CAD build for the part. Positions are in the model's coordinates, mm. Coordinates: 2 decimals unless noted, no trailing zeros. Order: outer loops, then holes, each group sorted by start corner. A loop starts at its lowest first (then second) coordinate and runs counter-clockwise, first axis right, second up. Notation, with made-up numbers: (28, -13.5) - (61, -13.5) arc R17 cw to (61, 19.5) - close; hole circle Ø2 at (4.25, 24.5). An arc over 180 degrees is marked (long way). Write each question's results on one line, items separated by ' | '. Start each with the question number.
Q1. Wall check: probe 1 along Z at (x, y) = (-81, -0.9); probe 2 along Z at (x, y) = (0, -1.25); probe 3 along X at (y, z) = (-0.85, 132). Give the ranges that are in metal, low to high.
Q2. Pin check, flat tips, straight feed: P1, Ø2.5, axis at x = 24.87, z = 21.07, coming from the +Y side; P2, Ø1.6, axis at y = -2.5, z = -1, coming from the +X side; P3, Ø1.1, axis at x = -4, y = -2.5, coming from the -Z side. Stop position of each tip, or through.
Q3. Band-saw the part on B-B, the plane x = 74.5. Write the cut outline in (y, z).
Q4. Pull direction X, two halves, no side cores. Call faces 1 (the flat face through (161.809, -1.878, 105.064)), 2 (the flat face through (58, -3.81, 54)), 3 (the flat face through (155.96, -1.88, 7.79)): released by +X, released by -X, zero draft, split by the parting line, or undercut.
Q5. Band-saw the part on A-A, the plane y = -0.9. Count the separate pieces of the cut face and the enclosed holes in it, then the cut area to 3 significant figures.
```python
from build123d import *

# Parameters (mm, degrees)
F0_R     = 1.5875
F1_DEPTH = 3.81


with BuildPart() as f1:
    # F0 (on Front) → F1 (new body)
    with BuildSketch(Plane.XZ):
        with BuildLine():
            Line((-43.090851702, -3.1242), (-43.090851702, 0))
            Line((-43.090851702, 0), (11.7375096306, 0))
            Line((11.7375096306, 0), (45.617762953, 11.4486236125))
            add(Edge.make_bspline(
                [(45.617762953, 11.4486236125), (43.9961000977, 8.6191003913), (40.3730056188, 4.577922731), (44.1195508196, 1.4224311064), (45.617762953, 0)],
                knots=[0, 0, 0, 0, 0.5388146408, 1, 1, 1, 1], degree=3))
            Line((45.617762953, 0), (77.7362398488, 0))
            Line((77.7362398488, 0), (77.7362398488, -3.1242))
            Line((77.7362398488, -3.1242), (103.1362398488, -3.1242))
            Line((103.1362398488, -3.1242), (103.1362398488, 0))
            Line((103.1362398488, 0), (137.1024620031, 0))
            Line((137.1024620031, 0), (175.3601329191, 15.8024989069))
            add(Edge.make_bspline(
                [(176.9877400097, 108.5755596732), (171.7473141945, 103.3597046798), (164.3550587217, 79.2093285896), (191.2164116111, 47.498469968), (169.6077040725, 23.5923640125), (175.3601329191, 15.8024989069)],
                knots=[0, 0, 0, 0, 0.3117132351, 0.6730053796, 1, 1, 1, 1], degree=3))
            Line((176.9877400097, 108.5755596732), (146.1987151904, 101.452911742))
            ThreePointArc((146.1987151904, 101.452911742), (91.5320388396, 140.0844195098), (36.3692378486, 102.1647111449))
            add(Edge.make_bspline(
                [(-15.078710516, 63.5241562685), (0.3297940237, 63.5041378405), (27.1279570327, 77.8387740817), (31.1426373051, 91.6452955028), (36.3692378486, 102.1647111449)],
                knots=[0, 0, 0, 0, 0.5551499724, 1, 1, 1, 1], degree=3))
            add(Edge.make_bspline(
                [(-15.078710516, 63.5241562685), (-30.8021855302, 63.8675037628), (-65.4962545936, 70.9878737096), (-114.1797542997, 45.7754396965), (-122.9711554478, 12.7121701485), (-144.690851702, 0)],
                knots=[0.2992076009, 0.2992076009, 0.2992076009, 0.2992076009, 0.50107299, 0.7437623527, 1, 1, 1, 1], degree=3))
            Line((-144.690851702, 0), (-68.490851702, 0))
            Line((-68.490851702, 0), (-68.490851702, -3.1242))
            Line((-68.490851702, -3.1242), (-43.090851702, -3.1242))
        make_face()
        with Locations((-80.1899433136, 10.7241785154)):
            Circle(F0_R, mode=Mode.SUBTRACT)
        with Locations((-45.4173433136, 19.2251093046)):
            Circle(F0_R, mode=Mode.SUBTRACT)
        with Locations((-20.6142470102, 17.4490999235)):
            Circle(F0_R, mode=Mode.SUBTRACT)
        with Locations((0, 21.0686270148)):
            Circle(F0_R, mode=Mode.SUBTRACT)
        with Locations((24.8666, 21.0686270148)):
            Circle(F0_R, mode=Mode.SUBTRACT)
        with Locations((139.4535154104, 10.7241785154)):
            Circle(F0_R, mode=Mode.SUBTRACT)
        with BuildLine():
            ThreePointArc((30.7592003997, 41.2713398651), (30.8999876678, 40.90769576), (30.9478799796, 40.5207016819))
            ThreePointArc((30.9478799796, 40.5207016819), (27.8207722914, 40.1337076037), (30.7592003997, 41.2713398651))
        make_face(mode=Mode.SUBTRACT)
        with BuildLine():
            ThreePointArc((65.9967244268, 59.3286920018), (64.796218505, 57.7890843136), (63.0104040067, 58.5780538185))
            ThreePointArc((63.0104040067, 58.5780538185), (63.5221237134, 60.6452057975), (65.6301646769, 60.3433156541))
            ThreePointArc((65.6301646769, 60.3433156541), (65.9022748106, 59.8680961189), (65.9967244268, 59.3286920018))
        make_face(mode=Mode.SUBTRACT)
        with BuildLine():
            ThreePointArc((92.7401996638, 81.553008482), (91.6921037808, 80.0599580982), (89.9317594137, 80.5383848296))
            ThreePointArc((89.9317594137, 80.5383848296), (90.6132955467, 83.0460588657), (92.7401996638, 81.553008482))
        make_face(mode=Mode.SUBTRACT)
    extrude(amount=F1_DEPTH)


solid = f1.part
```
Results below:
1) probe 1: z = 0 to 9.36, 12.09 to 60.77 | probe 2: z = 0 to 19.48, 22.66 to 65.89 | probe 3: x = 61.47 to 120.84
2) P1: passes through | P2: stops at x = 103.14 | P3: stops at z = 0
3) outline: (-3.81, 0) - (0, 0) - (0, 137.67) - (-3.81, 137.67) - close
4) face 1: undercut | face 2: zero draft | face 3: released by +X
5) separate pieces: 1 | enclosed holes: 9 | area: 27,000 mm²
